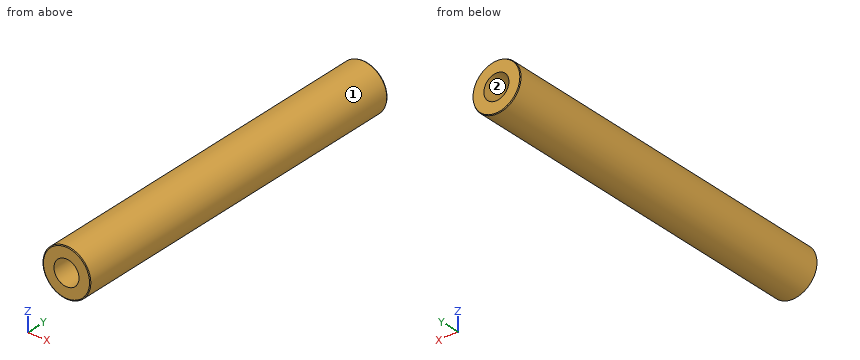
```python
from build123d import *
from OCP.BRepFilletAPI import BRepFilletAPI_MakeChamfer

# Parameters (mm, degrees)
SKETCH1_R           = 40
BOSS_EXTRUDE1_DEPTH = 600
SKETCH2_R           = 20.935503309
CUT_EXTRUDE1_DEPTH  = 603.660766933
CHAMFER1_SIZE       = 1.475151
CHAMFER1_SIZE2      = 0.851679


with BuildPart() as part:
    # Sketch1 → Boss-Extrude1 (new body)
    with BuildSketch(Plane(origin=(0, 0, 0), x_dir=(1, 0, 0), z_dir=(0, 1, 0))):
        with Locations(Location((0, 0, 0), (0, 0, 270))):
            Circle(SKETCH1_R)
    extrude(amount=BOSS_EXTRUDE1_DEPTH)

    # Sketch2 → Cut-Extrude1 (cut, through all)
    with BuildSketch(Plane(origin=(0, 0, 0), x_dir=(1, 0, 0), z_dir=(0, 1, 0))):
        with Locations(Location((0, 0, 0), (0, 0, 270))):
            Circle(SKETCH2_R)
    extrude(amount=CUT_EXTRUDE1_DEPTH, mode=Mode.SUBTRACT)

    # Chamfer1: one chamfer whose edges measure the first distance from different faces: ONE call of the kernel's chamfer builder (chamfer() names one face for all edges)
    chamfer1_edges_1 = [part.edges().sort_by_distance(p)[0] for p in [
        (0, 0, -40),
    ]]
    chamfer1_side_1 = [part.faces().sort_by_distance(p)[0] for p in [
        (0, 0, -38.86862915),
    ]]
    chamfer1_edges_2 = [part.edges().sort_by_distance(p)[0] for p in [
        (0, 600, -40),
    ]]
    chamfer1_side_2 = [part.faces().sort_by_distance(p)[0] for p in [
        (0, 300, -40),
    ]]
    chamfer1 = BRepFilletAPI_MakeChamfer(part.part.solid().wrapped)
    for e in chamfer1_edges_1:
        chamfer1.Add(CHAMFER1_SIZE, CHAMFER1_SIZE2, e.wrapped, chamfer1_side_1[0].wrapped)  # the first distance lies on this face
    for e in chamfer1_edges_2:
        chamfer1.Add(CHAMFER1_SIZE, CHAMFER1_SIZE2, e.wrapped, chamfer1_side_2[0].wrapped)  # the first distance lies on this face
    add(Compound.cast(chamfer1.Shape()), mode=Mode.REPLACE)


solid = part.part
```
CAD build for the part. Positions are in the model's coordinates, mm. Face numbers are marked on the shaded views. Give positions to 0.01 mm unless a question says otherwise; leave off trailing zeros. Loops run counter-clockwise (first coordinate to the right, second up) from the corner with the lowest first, then second, coordinate; pieces in that order, holes last. Notation, with made-up numbers: (13, 55.5) -> (47, 55.5) arc R30 cw to (47, 82.5) -> close; hole circle Ø7 at (45.25, -2). An arc over 180 degrees is marked (long way). Use a Markdown table: item, result.
1. Slice it at C-C (y = 386). List the corners of the cut face in (x, z).
Check result:
| item | result |
|---|---|
| outline | circle Ø80 at (0, 0); hole circle Ø41.87 at (0, 0) |
2. Mould opens along Z. For the marked faces 1 and 2 say: pulls with the +Z half, pulls with the -Z half, needs draft (parallel to the pull), parting line crosses it, or undercut.
Check result:
| item | result |
|---|---|
| face 1 | parting line crosses it |
| face 2 | undercut |
3. Slice it at A-A (x = 0). List the corners of the cut face in (y, z), plus the area to 3 significant figures.
Check result:
| item | result |
|---|---|
| outline | (0, -38.52) -> (0.85, -40) -> (598.52, -40) -> (600, -39.15) -> (600, -20.94) -> (0, -20.94) -> close; (0, 20.94) -> (600, 20.94) -> (600, 39.15) -> (598.52, 40) -> (0.85, 40) -> (0, 38.52) -> close |
| area | 22,900 mm^2 |
4. Slice it at B-B (z = 0). List the corners of the cut face in (x, y).
Check result:
| item | result |
|---|---|
| outline | (-40, 0.85) -> (-38.52, 0) -> (-20.94, 0) -> (-20.94, 600) -> (-39.15, 600) -> (-40, 598.52) -> close; (20.94, 0) -> (38.52, 0) -> (40, 0.85) -> (40, 598.52) -> (39.15, 600) -> (20.94, 600) -> close |
5. Wall check: L1, parallel to X at y = 456, z = 0; L2, parallel to Z at x = 2, y = 398.5; L3, parallel to Z at x = -14, y = 189.5. Give the ranges that are in metal, low to high. Write a range as [from, to].
Check result:
| item | result |
|---|---|
| L1 | x = [-40, -20.94], [20.94, 40] |
| L2 | z = [-39.95, -20.84], [20.84, 39.95] |
| L3 | z = [-37.47, -15.57], [15.57, 37.47] |
6. Flat gauge pins, fed straight in: pin 1 (5 mm diameter, centred on x = -19.5, y = 248, fed in from -Z); pin 2 (8 mm diameter, centred on x = 29.5, y = 360.5, fed in from +Z); pin 3 (1 mm diameter, centred on x = -13, z = 23.5, fed in from -Y); pin 4 (1.5 mm diameter, centred on x = -32, y = 392, fed in from +Z). Where does each tip first touch, or does it go through?
Check result:
| item | result |
|---|---|
| pin 1 | stops at z = -36.21 |
| pin 2 | stops at z = 30.82 |
| pin 3 | stops at y = 0 |
| pin 4 | stops at z = 24.97 |
